```python
from build123d import *

# Parameters (mm, degrees)
SKETCH_1_W          = 10
SKETCH_1_H          = 10
SKETCH_1_W_2        = 8
SKETCH_1_H_2        = 8
EXTRUDE_1_DEPTH     = 65
SKETCH_2_R          = 2.1
CUT_EXTRUDE_1_DEPTH = 60
SKETCH_3_R          = 2.1
CUT_EXTRUDE_2_DEPTH = 66.954529791


with BuildPart() as part:
    # 草图1 → 凸台-拉伸1 (new body)
    with BuildSketch(Plane.XY):
        Rectangle(SKETCH_1_W, SKETCH_1_H)
        Rectangle(SKETCH_1_W_2, SKETCH_1_H_2, mode=Mode.SUBTRACT)
    extrude(amount=EXTRUDE_1_DEPTH)

    # 草图2 → 切除-拉伸1 (cut)
    with BuildSketch(Plane(origin=(0, 5, 0), x_dir=(1, 0, 0), z_dir=(0, 1, 0))):
        with Locations(Location((0, -4.5, 0), (0, 0, 270))):
            Circle(SKETCH_2_R)
        with Locations(Location((0, -32.5, 0), (0, 0, 270))):
            Circle(SKETCH_2_R)
    cut_extrude_1 = extrude(amount=-CUT_EXTRUDE_1_DEPTH, mode=Mode.SUBTRACT)

    # 镜向1: 切除-拉伸1 across plane
    add(cut_extrude_1.mirror(Plane(origin=(0, 0, 32.5), x_dir=(1, 0, 0), z_dir=(0, 0, -1))), mode=Mode.SUBTRACT)

    # 草图3 → 切除-拉伸2 (cut, through all)
    with BuildSketch(Plane.ZY.offset(5)):
        with Locations(Location((12, 0, 0), (0, 0, 270))):
            Circle(SKETCH_3_R)
    cut_extrude_2 = extrude(amount=-CUT_EXTRUDE_2_DEPTH, mode=Mode.SUBTRACT)

    # 镜向2: 切除-拉伸2 across plane
    add(cut_extrude_2.mirror(Plane(origin=(0, 0, 32.5), x_dir=(1, 0, 0), z_dir=(0, 0, -1))), mode=Mode.SUBTRACT)


solid = part.part
```
Read the model definition and answer for the solid it produces. Units are mm, in the model's axes. A direction names the side the tool comes from. Give positions to 0.01 mm unless a question says otherwise; leave off trailing zeros. Order: outer loops, then holes, each group sorted by start corner. A loop starts at its lowest first (then second) coordinate and runs counter-clockwise, first axis right, second up.
(1) Straight lines are drawn through the part: L1, parallel to Y at x = -0.5, z = 7; L2, parallel to Y at x = -4.35, z = 53. For each, find the intervals that lie inside material, in ascending order.
(2) Find section B-B (y = 0). Give the vertices of the cut face in (x, z).
(3) Find section A-A (z = 23.5). Give the vertices of the cut face in (x, y).
(4) Find section D-D (z = 53). Give the vertices of the cut face in (x, y).
(5) For a pull along Y with two mould halves and no side action, classify faces 1 (the flat face through (-5, 0, 32)), 2 (the flat face through (-4, 0, 32)), 3 (the flat face through (2.2, -5, 32)) as released by +Y, released by -Y, zero draft, split by the parting line, or undercut.
(6) For faces 4 (the cylindrical face through (0.09, 4.51, 2.4)), 5 (the flat face through (4, 0, 32)), determine the directions among +Z, -Z, +X, -X, +Y, -Y from which every point of the face is accessible in a straight line to the end or side of a thin tool.
(7) Given pin 1 (3.5 mm diameter, centred on x = 0, z = 32.5, fed in from +Y); pin 2 (5 mm diameter, centred on y = 0, z = 12, fed in from -X), each flat-ended and moving along its own axis, determine where each tip first touches the part or whether it passes through.
(8) Find section C-C (x = 0). Give the number of separate pieces and of enclosed holes in the cut face, plus the area to 3 significant figures.
Result sheet:
1. L1: y = -5 to -4, 4 to 5
1. L2: y = -5 to -2.1, 2.1 to 5
2. outline: (-5, 0) - (-4, 0) - (-4, 9.9) - (-5, 9.9) - close; (-5, 14.1) - (-4, 14.1) - (-4, 50.9) - (-5, 50.9) - close; (-5, 55.1) - (-4, 55.1) - (-4, 65) - (-5, 65) - close; (4, 0) - (5, 0) - (5, 9.9) - (4, 9.9) - close; (4, 14.1) - (5, 14.1) - (5, 50.9) - (4, 50.9) - close; (4, 55.1) - (5, 55.1) - (5, 65) - (4, 65) - close
3. outline: (-5, -5) - (5, -5) - (5, 5) - (-5, 5) - close; hole (-4, -4) - (4, -4) - (4, 4) - (-4, 4) - close
4. outline: (-5, -5) - (5, -5) - (5, -2.1) - (4, -2.1) - (4, -4) - (-4, -4) - (-4, -2.1) - (-5, -2.1) - close; (-5, 2.1) - (-4, 2.1) - (-4, 4) - (4, 4) - (4, 2.1) - (5, 2.1) - (5, 5) - (-5, 5) - close
5. face 1: zero draft
5. face 2: undercut
5. face 3: released by -Y
6. face 4: +Y, -Y
6. face 5: +Z, -Z
7. pin 1: passes through
7. pin 2: stops at x = -5
8. separate pieces: 8
8. enclosed holes: 0
8. area: 105 mm2
